from build123d import *

# Parameters (mm, degrees)
SKETCH_2_R          = 1.5
CUT_EXTRUDE_1_DEPTH = 3
SKETCH_3_R          = 4.25
CUT_EXTRUDE_2_DEPTH = 18
SKETCH_6_R          = 1.25
EXTRUDE_1_DEPTH     = 6.5
SKETCH_7_R          = 23
EXTRUDE_2_DEPTH     = 1.6
SKETCH_10_R         = 1.25
EXTRUDE_3_DEPTH     = 5.5


with BuildPart() as part:
    # 草图1 → 旋转1 (revolve)
    with BuildSketch(Plane.XY, mode=Mode.PRIVATE) as revolve_1_sk:
        Polygon((23, 22.1), (0, 22.1), (0, 0), (4.75, 0), (7.5, 4.1), (22.5, 4.1), (22.5, 5.6), (23.5, 5.6), (23.5, 7.6), (22.5, 7.6), (22.5, 8.1), (23.5, 8.1), (23.5, 21.6), align=None)
    revolve(revolve_1_sk.sketch.rotate(Axis((0, 0, 0), (0, 1, 0)), 90), axis=Axis((0, 0, 0), (0, 1, 0)))

    # 草图2 → 切除-拉伸1 (cut)
    with BuildSketch(Plane(origin=(0, 22.1, 0), x_dir=(1, 0, 0), z_dir=(0, 1, 0))):
        with Locations(Location((0, 11, 0), (0, 0, 270))):
            Circle(SKETCH_2_R)
        with Locations(Location((11, 0, 0), (0, 0, 270))):
            Circle(SKETCH_2_R)
        with Locations(Location((0, -11, 0), (0, 0, 270))):
            Circle(SKETCH_2_R)
        with Locations(Location((-11, 0, 0), (0, 0, 270))):
            Circle(SKETCH_2_R)
    extrude(amount=-CUT_EXTRUDE_1_DEPTH, mode=Mode.SUBTRACT)

    # 草图3 → 切除-拉伸2 (cut)
    with BuildSketch(Plane(origin=(0, 22.1, 0), x_dir=(1, 0, 0), z_dir=(0, 1, 0))):
        with Locations(Location((0, 0, 0), (0, 0, 270))):
            Circle(SKETCH_3_R)
    extrude(amount=-CUT_EXTRUDE_2_DEPTH, mode=Mode.SUBTRACT)

    # 草图6 → 凸台-拉伸1 (add)
    with BuildSketch(Plane.XZ.offset(-4.1)):
        with Locations(Location((0, 19.25, 0), (0, 0, 90))):
            Circle(SKETCH_6_R)
        with Locations(Location((19.25, 0, 0), (0, 0, 90))):
            Circle(SKETCH_6_R)
        with Locations(Location((0, -19.25, 0), (0, 0, 90))):
            Circle(SKETCH_6_R)
        with Locations(Location((-19.25, 0, 0), (0, 0, 90))):
            Circle(SKETCH_6_R)
    extrude(amount=EXTRUDE_1_DEPTH)

    # 草图7 → 凸台-拉伸2 (add)
    with BuildSketch(Plane.XZ.offset(2.4)):
        with Locations(Location((0, 0, 0), (0, 0, 270))):
            Circle(SKETCH_7_R)
    extrude(amount=EXTRUDE_2_DEPTH)

    # 草图10 → 凸台-拉伸3 (add)
    with BuildSketch(Plane.XZ.offset(4)):
        with Locations(Location((0, 19.25, 0), (0, 0, 90))):
            Circle(SKETCH_10_R)
        with Locations(Location((19.25, 0, 0), (0, 0, 90))):
            Circle(SKETCH_10_R)
        with Locations(Location((0, -19.25, 0), (0, 0, 90))):
            Circle(SKETCH_10_R)
        with Locations(Location((-19.25, 0, 0), (0, 0, 90))):
            Circle(SKETCH_10_R)
    extrude(amount=EXTRUDE_3_DEPTH)


solid = part.part
Model file for the job. Use its own axes, mm. A direction names the side the tool comes from. Coordinates: 2 decimals unless noted, no trailing zeros. Order: outer loops, then holes, each group sorted by start corner. A loop starts at its lowest first (then second) coordinate and runs counter-clockwise, first axis right, second up. Notation, with made-up numbers: M 88.5,50 L 145.5,50 A24 cw 145.5,85 Z; hole C -19.75,-32 d5. An arc over 180 degrees is marked long. Return JSON: item names as keys, results as strings.
1. Saw through at C-C (y = 10). Give the cut face in (x, z).
Ans:
{"outline": "C 0,0 d47; hole C 0,0 d8.5"}
2. Flat gauge pins, fed straight in: pin 1 (5 mm diameter, centred on x = 10.5, y = 10.5, fed in from -Z); pin 2 (6 mm diameter, centred on x = 10.5, y = 5, fed in from -Z); pin 3 (0.9 mm diameter, centred on x = 0.5, z = -11, fed in from +Y); pin 4 (4 mm diameter, centred on x = 12.5, y = 0.5, fed in from +Z). Where does each tip first touch, or does it go through?
Ans:
{"pin 1": "z = -22.1", "pin 2": "z = -22.25", "pin 3": "y = 19.1", "pin 4": "through"}
3. Saw through at B-B (y = 1.5). Give the cut face in (x, z).
Ans:
{"outline": "C -19.25,0 d2.5; C 0,0 d11.51; C 0,-19.25 d2.5; C 0,19.25 d2.5; C 19.25,0 d2.5"}
4. Tool access for faces 1 (the face through (0, 7.6, -23)), 2 (the face through (0.07, 20.62, -12.5)), 3 (the face through (-19, -9.5, 0)), 4 (the face through (19.394, -3.189, -12.365)): list every direction of +Z, -Z, +X, -X, +Y, -Y with a clear straight run to the whole face (end or side of a thin tool).
Ans:
{"face 1": "none", "face 2": "+Y", "face 3": "+Z, -Z, +X, -X, -Y", "face 4": "-Y"}
5. Pull direction Y, two halves, no side cores. Call faces 5 (the face through (0, 0, 0)), 6 (the face through (0, 1, -18)), 7 (the face through (11, 19.1, 0)), 8 (the face through (0, -9.5, 19)): +Y half, -Y half, draft (parallel to the pull), parting line (faces both ways), or undercut.
Ans:
{"face 5": "undercut", "face 6": "undercut", "face 7": "+Y half", "face 8": "-Y half"}
6. Saw through at A-A (y = 20.5). Give the cut face in (x, z).
Ans:
{"outline": "C 0,0 d47; hole C -11,0 d3; hole C 0,0 d8.5; hole C 0,-11 d3; hole C 0,11 d3; hole C 11,0 d3"}
7. Drill centre lines: probe 1 along X at (y, z) = (21.25, 0); probe 2 along Y at (x, z) = (9, -16); probe 3 along X at (y, z) = (20, -1). Where is each one in solid material? Low to high.
Ans:
{"probe 1": "-23.5 to -12.5, -9.5 to -4.25, 4.25 to 9.5, 12.5 to 23.5", "probe 2": "-4 to -2.4, 4.1 to 22.1", "probe 3": "-23.48 to -12.12, -9.88 to -4.13, 4.13 to 9.88, 12.12 to 23.48"}
